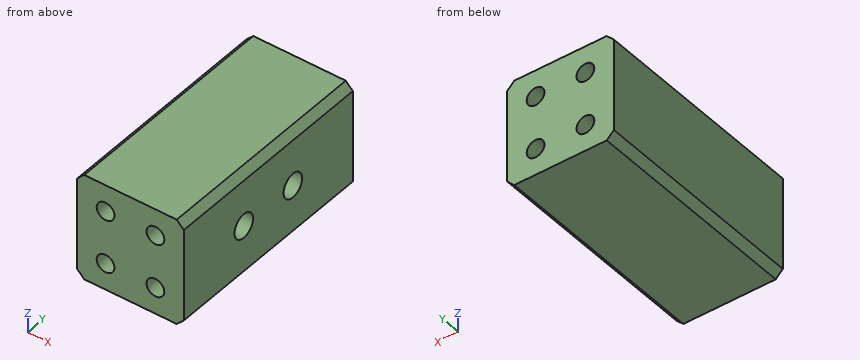
```python
from build123d import *

# Parameters (mm, degrees)
F0_W     = 30
F0_H     = 30
F1_DEPTH = 62
F3_D     = 5
F3_DEPTH = 20
F3_TIP   = 1.5021515476
F5_D     = 6.8
F5_DEPTH = 20
F5_TIP   = 2.0429261047
F7_D     = 5
F7_DEPTH = 20
F7_TIP   = 1.5021515476
F8_SIZE  = 2


with BuildPart() as f1:
    # F0 (on Front) → F1 (new body)
    with BuildSketch(Plane.XZ):
        with Locations((2.5945728272, 3.4459190071)):
            Rectangle(F0_W, F0_H)
    extrude(amount=F1_DEPTH)

    # F3
    with Locations(Plane.XZ.offset(62)):
        with Locations((-4.4054271728, 10.9459190071), (9.5945728272, 10.9459190071), (9.5945728272, -4.0540809929), (-4.4054271728, -4.0540809929)):
            Hole(F3_D / 2, depth=F3_DEPTH)
            with Locations((0, 0, -(F3_DEPTH + F3_TIP / 2))):  # 118° drill point
                Cone(0, F3_D / 2, F3_TIP, mode=Mode.SUBTRACT)

    # F5
    with Locations(Plane.YZ.offset(17.5945728272)):
        with Locations((-40, 3.4459190071), (-22, 3.4459190071)):
            Hole(F5_D / 2, depth=F5_DEPTH)
            with Locations((0, 0, -(F5_DEPTH + F5_TIP / 2))):  # 118° drill point
                Cone(0, F5_D / 2, F5_TIP, mode=Mode.SUBTRACT)

    # F7
    with Locations(Plane(origin=(0, 0, 0), x_dir=(-1, 0, 0), z_dir=(0, 1, 0))):
        with Locations((-9.5945728272, 10.9459190071), (4.4054271728, 10.9459190071), (4.4054271728, -4.0540809929), (-9.5945728272, -4.0540809929)):
            Hole(F7_D / 2, depth=F7_DEPTH)
            with Locations((0, 0, -(F7_DEPTH + F7_TIP / 2))):  # 118° drill point
                Cone(0, F7_D / 2, F7_TIP, mode=Mode.SUBTRACT)

    # F8
    f8_edges = [f1.edges().sort_by_distance(p)[0] for p in [
        (-12.405427, -31, 18.445919),
        (17.594573, -31, 18.445919),
        (17.594573, -31, -11.554081),
        (-12.405427, -31, -11.554081),
    ]]
    chamfer(f8_edges, length=F8_SIZE)


solid = f1.part
```
Input: part model. Units: mm. Frame: model coordinates. Give positions to 0.01 mm unless a question says otherwise; leave off trailing zeros. Write each loop counter-clockwise with the first axis right and the second up, starting at its lowest first coordinate (ties: lowest second). Pieces come first, ordered by that corner, then holes. Notation, with made-up numbers: (18, 44) - (48, 44) arc R22 ccw to (48, 67) - close; hole circle Ø9 at (-31.5, 0). An arc over 180 degrees is marked (long way). Write item = value, one per line. Start each with the question number.
1) Material intervals for L1, parallel to Z at x = -4.25, y = -47; L2, parallel to X at y = -9, z = -3.75; L3, parallel to Z at x = -6.5, y = -3, sorted ascending. Write a range as [from, to].
2) Cut plane A-A (y = -12). Return loops of the section in (x, z).
3) Cut plane B-B (x = 14). Return loops of the section in (y, z), and give its area (3 significant figures).
4) Pin query (flat end, axial travel): pin 1 (4.5 mm diameter, centred on x = 9.59, z = -4.05, fed in from +Y); pin 2 (4.5 mm diameter, centred on x = -4.41, z = 10.95, fed in from -Y); pin 3 (3 mm diameter, centred on x = 9.59, z = -4.05, fed in from +Y); pin 4 (10 mm diameter, centred on x = 10.5, z = 0, fed in from +Y). Return the tip coordinate at first contact, or that it passes through.
Answers follow:
q1.L1 = [-11.55, -6.55], [-1.56, 8.45], [13.44, 18.45]
q1.L2 = [-12.41, -6.89], [-1.92, 7.11], [12.08, 17.59]
q1.L3 = [-11.55, -5.42], [-2.69, 9.58], [12.31, 18.45]
q2.outline = (-12.41, -9.55) - (-10.41, -11.55) - (15.59, -11.55) - (17.59, -9.55) - (17.59, 16.45) - (15.59, 18.45) - (-10.41, 18.45) - (-12.41, 16.45) - close; hole circle Ø5 at (-4.41, -4.05); hole circle Ø5 at (-4.41, 10.95); hole circle Ø5 at (9.59, -4.05); hole circle Ø5 at (9.59, 10.95)
q3.outline = (-62, -11.55) - (0, -11.55) - (0, 18.45) - (-62, 18.45) - close; hole circle Ø6.8 at (-40, 3.45); hole circle Ø6.8 at (-22, 3.45)
q3.area = 1,790 mm^2
q4.pin_1 = -20.15
q4.pin_2 = -41.85
q4.pin_3 = -20.6
q4.pin_4 = 0
